For this review, take the finished solid that the model builds, in its own axes (mm). Face numbers are marked on the shaded views. A direction names the side the tool comes from. Round coordinates to 2 decimals unless told otherwise and drop trailing zeros. Loops run counter-clockwise (first coordinate to the right, second up) from the corner with the lowest first, then second, coordinate; pieces in that order, holes last.
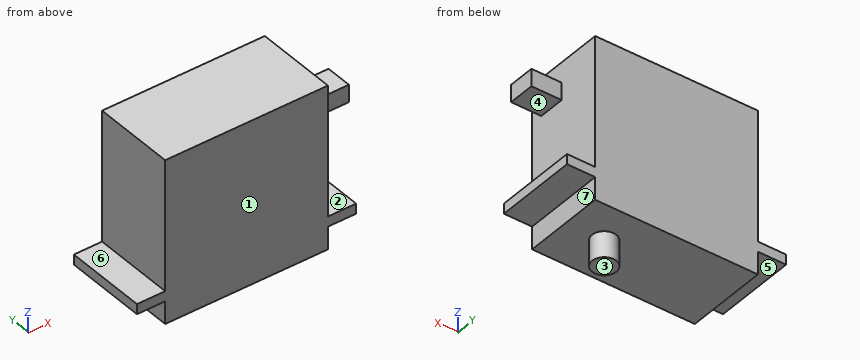
```python
from build123d import *

# Parameters (mm, degrees)
SKETCH2_W           = 7
SKETCH2_H           = 2.5
BOSS_EXTRUDE3_DEPTH = 20.5
SKETCH4_W           = 4.3
SKETCH4_H           = 6.6
WIRE_2_DEPTH        = 7.5
SKETCH6_R           = 3
BOSS_EXTRUDE5_DEPTH = 6.4


with BuildPart() as part:
    # Sketch2 → Boss-Extrude3 (new body)
    with BuildSketch(Plane(origin=(0, 0, 0), x_dir=(1, 0, 0), z_dir=(0, 1, 0))):
        with Locations((-26.15465113, 5.213732574)):
            Rectangle(SKETCH2_W, SKETCH2_H)
        Polygon((-2.45465113, -28.336267426), (-2.45465113, 12.063732574), (-22.65465113, 12.063732574), (-22.65465113, 6.463732574), (-22.65465113, 3.963732574), (-22.65465113, -28.336267426), align=None)
        Polygon((17.74534887, 12.063732574), (-2.45465113, 12.063732574), (-2.45465113, -28.336267426), (17.74534887, -28.336267426), (17.74534887, 3.963732574), (17.74534887, 6.463732574), align=None)
        with Locations((21.24534887, 5.213732574)):
            Rectangle(SKETCH2_W, SKETCH2_H)
    extrude(amount=BOSS_EXTRUDE3_DEPTH)

    # Sketch4 → Wire 2 (add)
    with BuildSketch(Plane(origin=(17.74534887, 0, 0), x_dir=(0, 0, -1), z_dir=(1, 0, 0))):
        with Locations((-21.186267426, 6.3)):
            Rectangle(SKETCH4_W, SKETCH4_H)
    extrude(amount=WIRE_2_DEPTH)

    # Sketch6 → Boss-Extrude5 (add)
    with BuildSketch(Plane(origin=(0, 0, -12.063732574), x_dir=(-1, 0, 0), z_dir=(0, 0, -1))):
        with Locations((-8.24534887, 11)):
            Circle(SKETCH6_R)
    extrude(amount=BOSS_EXTRUDE5_DEPTH)


solid = part.part
```
(1) Insertion check: pin 1 Ø3 at (x, z) = (16, -7.5) entering from -Y; pin 2 Ø2 at (x, y) = (-27, 8) entering from -Z; pin 3 Ø3 at (y, z) = (13.5, -5.5) entering from +X; pin 4 Ø1.7 at (y, z) = (13, -10.5) entering from -X. Each pin has a flat end and moves straight along its axis. Give the tip position at first contact, or say it passes through.
(2) Add section A-A (y = 15.75). Give the boundary of the cut face in (x, z).
(3) The part is to be moulded in two halves that separate along Z. For the marked faces 1, 2 and 3, say which applies: pulls with the +Z half, pulls with the -Z half, needs draft (parallel to the pull), parting line crosses it, or undercut.
(4) Add section C-C (y = 11). Give the boundary of the cut face in (x, z).
(5) For the marked faces 4, 5, 6 and 7, list the 3-axis set-ups (+Z, -Z, +X, -X, +Y, -Y) from which the entire face can be reached by the end or side of a thin tool; tool diameter is ignored.
(6) Add section B-B (x = 17). Give the boundary of the cut face in (y, z).
(7) For L1, parallel to X at y = 14, z = -5.5; L2, parallel to Z at x = -3.5, y = 2.25; L3, parallel to X at y = 9.75, z = 9.5, list the stretches that pass through material, from the lowest coordinate up.
(8) Add section D-D (z = 1.5). Give the boundary of the cut face in (x, y), plus the area to 3 significant figures.
Outcome:
1. pin 1: stops at y = 0
1. pin 2: stops at z = -6.46
1. pin 3: stops at x = 24.75
1. pin 4: stops at x = -22.65
2. outline: (-29.65, -6.46) - (-22.65, -6.46) - (-22.65, -12.06) - (17.75, -12.06) - (17.75, -6.46) - (24.75, -6.46) - (24.75, -3.96) - (17.75, -3.96) - (17.75, 28.34) - (-22.65, 28.34) - (-22.65, -3.96) - (-29.65, -3.96) - close
3. face 1: needs draft
3. face 2: undercut
3. face 3: pulls with the -Z half
4. outline: (-29.65, -6.46) - (-22.65, -6.46) - (-22.65, -12.06) - (5.25, -12.06) - (5.25, -18.46) - (11.25, -18.46) - (11.25, -12.06) - (17.75, -12.06) - (17.75, -6.46) - (24.75, -6.46) - (24.75, -3.96) - (17.75, -3.96) - (17.75, 28.34) - (-22.65, 28.34) - (-22.65, -3.96) - (-29.65, -3.96) - close
5. face 4: +X, +Y, -Y
5. face 5: -Z, -X, +Y, -Y
5. face 6: +Z, -X, +Y, -Y
5. face 7: -Z, +X, +Y, -Y
6. outline: (0, -12.06) - (20.5, -12.06) - (20.5, 28.34) - (0, 28.34) - close
7. L1: x = -29.65 to 24.75
7. L2: z = -12.06 to 28.34
7. L3: x = -22.65 to 17.75
8. outline: (-22.65, 0) - (17.75, 0) - (17.75, 20.5) - (-22.65, 20.5) - close
8. area: 828 mm2
